from build123d import *

# Parameters (mm, degrees)
SKETCH_1_R      = 19
SKETCH_1_R_2    = 16
EXTRUDE_1_DEPTH = 6
FILLET_1_R      = 0.8
FILLET_2_R      = 0.5
FILLET_3_R      = 0.5


# Read off the part's stored shape, not the designer's step: 压凹1
with BuildPart() as part:
    # 草图1 → 凸台-拉伸1 (new body)
    with BuildSketch(Plane(origin=(0, 0, 0), x_dir=(1, 0, 0), z_dir=(0, 1, 0))):
        with Locations(Location((0, 0, 0), (0, 0, 270))):
            Circle(SKETCH_1_R)
        with Locations(Location((0, 0, 0), (0, 0, 270))):
            Circle(SKETCH_1_R_2, mode=Mode.SUBTRACT)
    extrude(amount=EXTRUDE_1_DEPTH)

    # 压凹1 outline → 压凹1 (revolve, cut)
    with BuildSketch(Plane.XY):
        with BuildLine():
            Line((16, 5), (16, 1))
            ThreePointArc((16, 1), (17, 3), (16, 5))
        make_face()
    revolve(axis=Axis((0, 0, 0), (0, 1, 0)), mode=Mode.SUBTRACT)

    # 圆角1
    fillet_1_edges = [part.edges().sort_by_distance(p)[0] for p in [
        (0, 0, -19),
        (0, 6, -19),
    ]]
    fillet(fillet_1_edges, radius=FILLET_1_R)

    # 圆角2
    fillet_2_edges = [part.edges().sort_by_distance(p)[0] for p in [
        (0, 0, -16),
    ]]
    fillet(fillet_2_edges, radius=FILLET_2_R)

    # 圆角3
    fillet_3_edges = [part.edges().sort_by_distance(p)[0] for p in [
        (0, 6, -16),
    ]]
    fillet(fillet_3_edges, radius=FILLET_3_R)


solid = part.part
The model under review builds one solid part; all positions refer to its coordinate system, in mm. Round coordinates to 2 decimals unless told otherwise and drop trailing zeros. Loops run counter-clockwise (first coordinate to the right, second up) from the corner with the lowest first, then second, coordinate; pieces in that order, holes last. Notation, with made-up numbers: (81, 27.25) -> (117, 27.25) arc R21 ccw to (117, 64.25) -> close; hole circle Ø2 at (-39.5, 47.25). An arc over 180 degrees is marked (long way). Answer as CSV lines item,"result".
1) To check wall thickness, follow line 1 along X through (y, z) = (5.25, 0); line 2 along Z through (x, y) = (-4, 2.2); line 3 along Y through (x, z) = (-4.5, -16). State the ranges of each line that lie inside material, in increasing order. Write a range as from..to.
Geometry results:
line 1,"x = -19..-16, 16..19"
line 2,"z = -18.57..-16.39, 16.39..18.57"
line 3,"y = 0..1.68, 4.32..6"
2) For P1, Ø2, axis at y = 4.5, z = -14.5, coming from the -X side; P2, Ø3, axis at x = -3.5, y = 3, coming from the -Z side; P3, Ø1, axis at x = -3, y = 3, coming from the +Z side, all flat-tipped, find the tip position at first contact; note any pin that passes through.
Geometry results:
P1,"stops at x = -13.37"
P2,"stops at z = -18.89"
P3,"stops at z = 18.83"
3) Add section A-A on z = 0. Write out the cut boundary in (x, y), plus the area to 3 significant figures.
Geometry results:
outline,"(-19, 0.8) arc R0.8 ccw to (-18.2, 0) -> (-16.5, 0) arc R0.5 ccw to (-16, 0.5) -> (-16, 1) arc R2.5 cw to (-16, 5) -> (-16, 5.5) arc R0.5 ccw to (-16.5, 6) -> (-18.2, 6) arc R0.8 ccw to (-19, 5.2) -> close; (16, 0.5) arc R0.5 ccw to (16.5, 0) -> (18.2, 0) arc R0.8 ccw to (19, 0.8) -> (19, 5.2) arc R0.8 ccw to (18.2, 6) -> (16.5, 6) arc R0.5 ccw to (16, 5.5) -> (16, 5) arc R2.5 cw to (16, 1) -> close"
area,"29.6 mm²"
4) Add section B-B on y = 4.4. Write out the cut boundary in (x, z).
Geometry results:
outline,"circle Ø38 at (0, 0); hole circle Ø33.14 at (0, 0)"
5) Draft analysis for pull direction Z (two halves, no side actions). For faces 1 (the face through (-6.13, 0.75, 14.78)), 2 (the face through (-6.13, 5.25, 14.78)), 3 (the face through (-15, 6, 8)), 4 (the face through (-11.56, 2.97, -15.08)), state which applies: pulls with the +Z half, pulls with the -Z half, needs draft (parallel to the pull), parting line crosses it, or undercut.
Geometry results:
face 1,"undercut"
face 2,"undercut"
face 3,"needs draft"
face 4,"parting line crosses it"
